from build123d import *

# Parameters (mm, degrees)
SCHIZZO1_R                   = 110
SCHIZZO1_R_2                 = 75.5
ESTRUSIONE_ESTRUSIONE1_DEPTH = 0.1
SCHIZZO3_R                   = 4.5
TAGLIO_ESTRUSIONE1_DEPTH     = 156.563524002


with BuildPart() as part:
    # Schizzo1 → Estrusione-Estrusione1 (new body)
    with BuildSketch(Plane.XY):
        Circle(SCHIZZO1_R)
        Circle(SCHIZZO1_R_2, mode=Mode.SUBTRACT)
    extrude(amount=ESTRUSIONE_ESTRUSIONE1_DEPTH)

    # Schizzo3 → Taglio-Estrusione1 (cut, through all)
    with BuildSketch(Plane.XY.offset(0.1)):
        with Locations((-65.40737726, 65.40737726)):
            Circle(SCHIZZO3_R)
        with Locations((65.40737726, 65.40737726)):
            Circle(SCHIZZO3_R)
        with Locations((65.40737726, -65.40737726)):
            Circle(SCHIZZO3_R)
        with Locations((-65.40737726, -65.40737726)):
            Circle(SCHIZZO3_R)
    extrude(amount=-TAGLIO_ESTRUSIONE1_DEPTH, mode=Mode.SUBTRACT)


solid = part.part
Source: CAD feature listing. Evaluate the final solid. Frame: model axes, mm. Give positions to 0.01 mm unless a question says otherwise; leave off trailing zeros. Order: outer loops, then holes, each group sorted by start corner. A loop starts at its lowest first (then second) coordinate and runs counter-clockwise, first axis right, second up. Notation, with made-up numbers: (51.25, 56.5) -> (87.25, 56.5) arc R17 ccw to (87.25, 67.5) -> close; hole circle Ø5 at (31.25, 2). An arc over 180 degrees is marked (long way). Write item = value, one per line.
Q1. Cut plane B-B, the plane x = -17. Output: boundary loops of the cut face in (y, z).
Data:
outline = (-108.68, 0) -> (-73.56, 0) -> (-73.56, 0.1) -> (-108.68, 0.1) -> close; (73.56, 0) -> (108.68, 0) -> (108.68, 0.1) -> (73.56, 0.1) -> close
Q2. Cut plane A-A, the plane y = 0. Output: boundary loops of the cut face in (x, z), and give its area (3 significant figures).
Data:
outline = (-110, 0) -> (-75.5, 0) -> (-75.5, 0.1) -> (-110, 0.1) -> close; (75.5, 0) -> (110, 0) -> (110, 0.1) -> (75.5, 0.1) -> close
area = 6.90 mm^2
Q3. Material intervals for line 1 (X direction, y = -23.5, z = 0.05); line 2 (Y direction, x = -37.5, z = 0.05); line 3 (X direction, y = 97, z = 0.05), sorted ascending. Write a range as from..to.
Data:
line_1 = -107.46..-71.75, 71.75..107.46
line_2 = -103.41..-65.53, 65.53..103.41
line_3 = -51.87..51.87
Q4. Pin query (flat end, axial travel): pin 1 (5.5 mm diameter, centred on x = -65.41, y = -65.41, fed in from -Z). Return the tip coordinate at first contact, or that it passes through.
Data:
pin_1 = through
